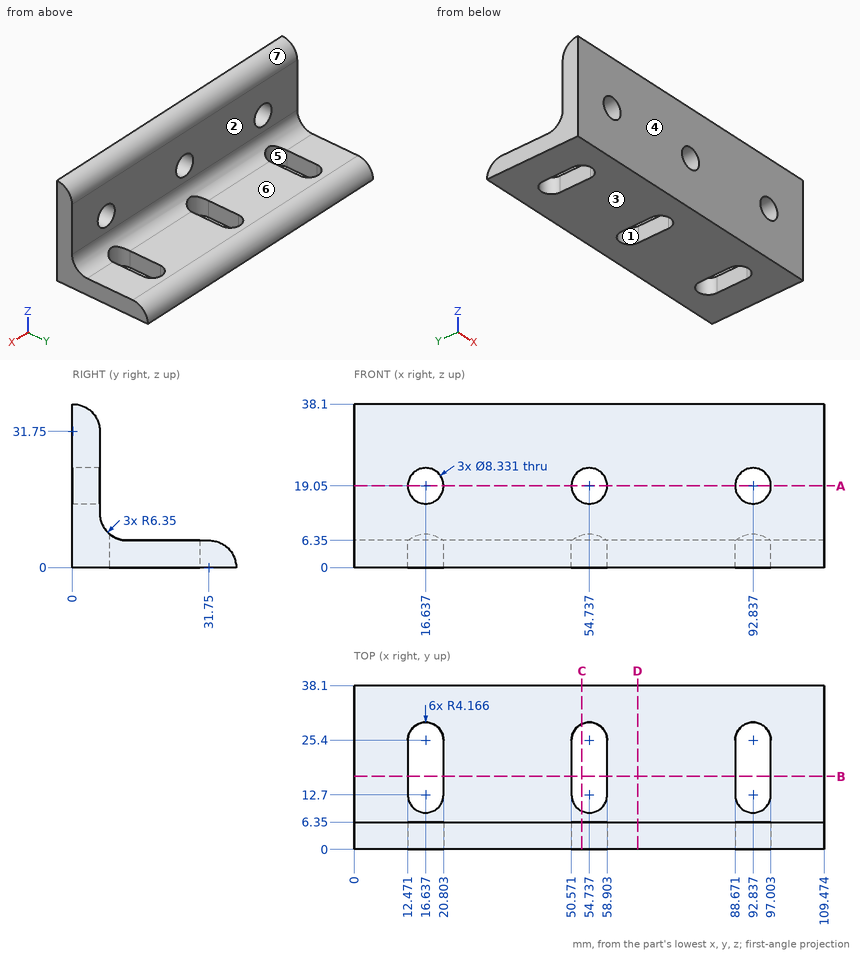
Here's the drawing with two shaded views (mm, measured from the low corner). I have some questions. A direction names the side the tool comes from. Coordinates: 2 decimals unless noted, no trailing zeros. Order: outer loops, then holes, each group sorted by start corner. A loop starts at its lowest first (then second) coordinate and runs counter-clockwise, first axis right, second up. Notation, with made-up numbers: (84.25, 77.5) - (130.25, 77.5) arc R27 cw to (130.25, 102.5) - close; hole circle Ø4 at (-20.5, 29.5). An arc over 180 degrees is marked (long way). Answer in a Markdown table with one row per item.
1. Suppose I cut it at D-D (x = 66). Please give me the cut outline in (y, z), and give its area (3 significant figures).
Reply:
| item | result |
|---|---|
| outline | (0, 0) - (38.1, 0) arc R6.35 ccw to (31.75, 6.35) - (12.7, 6.35) arc R6.35 cw to (6.35, 12.7) - (6.35, 31.75) arc R6.35 ccw to (0, 38.1) - close |
| area | 435 mm^2 |
2. If we mould it in two halves opening along Y, with no side actions, what happens to the marked faces 4, 5, 6 and 7? For each: pulls with the +Y half, pulls with the -Y half, needs draft (parallel to the pull), parting line crosses it, or undercut.
Reply:
| item | result |
|---|---|
| face 4 | pulls with the -Y half |
| face 5 | undercut |
| face 6 | needs draft |
| face 7 | pulls with the +Y half |
3. For pin 1 (9.5 mm diameter, centred on x = 54.737, z = 19.05, fed in from -Y); pin 2 (5 mm diameter, centred on x = 32.5, y = 27.5, fed in from +Z); pin 3 (15 mm diameter, centred on x = 69.5, z = 23, fed in from +Y); pin 4 (6.5 mm diameter, centred on x = 92.837, z = 19.05, fed in from +Y), each with a flat end and sliding along its axis, tell me the tip position at first contact or that it passes through.
Reply:
| item | result |
|---|---|
| pin 1 | stops at y = 0 |
| pin 2 | stops at z = 6.35 |
| pin 3 | stops at y = 6.35 |
| pin 4 | passes through |
4. For the marked faces 1, 2 and 3, which set-ups out of +Z, -Z, +X, -X, +Y, -Y let a thin tool reach every point of the face, with its end or its side?
Reply:
| item | result |
|---|---|
| face 1 | +Z, -Z |
| face 2 | +Z, +X, -X, +Y |
| face 3 | -Z, +X, -X, +Y, -Y |
5. If I drill on line 1 along X through (y, z) = (2, 19.05); line 2 along Y through (x, z) = (17, 29), over which ranges is the centre line in solid material (lowest first)?
Reply:
| item | result |
|---|---|
| line 1 | x = 0 to 12.47, 20.8 to 50.57, 58.9 to 88.67, 97 to 109.47 |
| line 2 | y = 0 to 6.35 |
6. Suppose I cut it at C-C (x = 53). Please give me the cut outline in (y, z).
Reply:
| item | result |
|---|---|
| outline | (0, 0) - (8.91, 0) - (8.91, 7.6) arc R6.35 cw to (6.35, 12.7) - (6.35, 15.26) - (0, 15.26) - close; (0, 22.84) - (6.35, 22.84) - (6.35, 31.75) arc R6.35 ccw to (0, 38.1) - close; (29.19, 0) - (38.1, 0) arc R6.35 ccw to (31.75, 6.35) - (29.19, 6.35) - close |
7. Suppose I cut it at A-A (z = 19.05). Please give me the cut outline in (x, y).
Reply:
| item | result |
|---|---|
| outline | (0, 0) - (12.47, 0) - (12.47, 6.35) - (0, 6.35) - close; (20.8, 0) - (50.57, 0) - (50.57, 6.35) - (20.8, 6.35) - close; (58.9, 0) - (88.67, 0) - (88.67, 6.35) - (58.9, 6.35) - close; (97, 0) - (109.47, 0) - (109.47, 6.35) - (97, 6.35) - close |
